Autodesk Inventor part; units mm, degrees
ref_plane "YZ Plane" through (0, 0, 0) normal (1, 0, 0) x (0, 1, 0)
ref_plane "XZ Plane" through (0, 0, 0) normal (0, 1, 0) x (-1, 0, 0)
ref_plane "XY Plane" through (0, 0, 0) normal (0, 0, 1) x (1, 0, 0)
sketch "Sketch1" plane through (0, 0, 0) normal (0, 0, 1) x (1, 0, 0)
  line L0 (-8.2268, 11.9764) -> (-8.2268, -9.0421)
  line L1 (-8.2268, -9.0421) -> (4.4732, -9.0421)
  line L2 (4.4732, -9.0421) -> (4.4732, 11.9764)
  line L3 (4.4732, 11.9764) -> (1.2982, 11.9764)
  line L4 (-8.2268, 11.9764) -> (-5.0518, 11.9764)
  line L5 (-5.0518, 11.9764) -> (-5.0518, 11.5954)
  line L6 (1.2982, 11.9764) -> (1.2982, 11.5954)
  arc A0 (-5.0518, 11.5954) -> (1.2982, 11.5954) centre (-1.8768, 11.5954) ccw
  dimension "d0" = 3.175
  dimension "d1" = 12.7
  dimension "d2" = 0.381
  dimension "d5" = 20.6375
  dimension "d6" = 3.175
  dimension "d7" = 21.0185
revolve "Revolution1" add sketch "Sketch1" angle 360 about axis through (-8.2268, -9.0421, 0) along (1, 0, 0)
sketch "Sketch2" plane through (4.4732, -9.0421, 0) normal (1, 0, 0) x (0, 0, -1)
  circle A0 centre (0, 0) radius 21.0185
hole "Hole1" at (4.4732, -9.0421, 0) direction (-1, 0, 0) diameter 9.525 end through all
sketch "Sketch3" plane through (4.4732, -9.0421, 0) normal (1, 0, 0) x (0, 0, -1)
  circle A0 centre (0, 0) radius 4.7625
  circle A1 centre (0, 0) radius 21.0185
  circle A2 centre (0, 0) radius 4.7625
  circle A3 centre (0, 0) radius 7.9375
  dimension "d15" = 3.175
extrude "Extrusion1" add sketch "Sketch3" along normal blind 12.7 contours A3
properties part number "pulley 1.5"
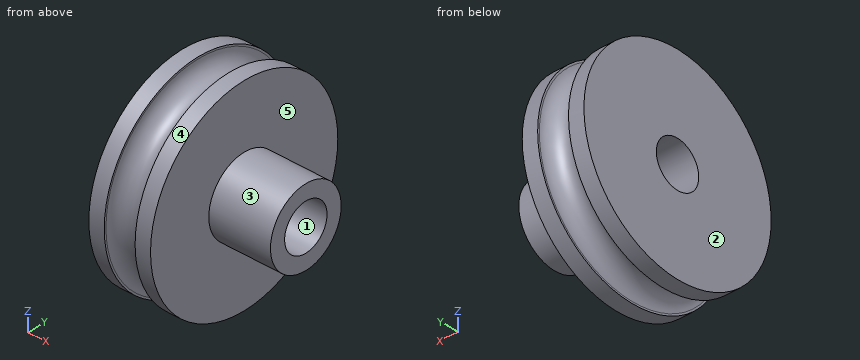
Read the model definition and answer for the solid it produces. Units are mm, in the model's axes. Face numbers are marked on the shaded views. A direction names the side the tool comes from. Round coordinates to 2 decimals unless told otherwise and drop trailing zeros. Write each loop counter-clockwise with the first axis right and the second up, starting at its lowest first coordinate (ties: lowest second). Pieces come first, ordered by that corner, then holes.
1. The part is cut by section A-A, the plane z = 0. Determine the outline of the cut face in (x, y) (3 decimals), then the cut area to 3 significant figures.
2. Straight lines are drawn through the part: L1, parallel to X at y = 1, z = 18; L2, parallel to X at y = -19, z = 8; L3, parallel to Y at x = 8.5, z = 0. For each, find the intervals that lie inside material, in ascending order.
3. Determine the mould class of the marked faces 1, 2 and 3 for opening direction Y: pulls with the +Y half, pulls with the -Y half, needs draft (parallel to the pull), parting line crosses it, or undercut.
4. The part is cut by section C-C, the plane x = 3.5. Determine the outline of the cut face in (y, z) (1 decimal), then the cut area to 3 significant figures.
5. The part is cut by section B-B, the plane x = 14.75. Determine the outline of the cut face in (y, z) (1 decimal).
6. Which of the six approach directions +Z, -Z, +X, -X, +Y, -Y give full straight-line access (tool end or side, diameter ignored) to the marked faces 4 and 5?
7. Given pin 1 Ø5 at (y, z) = (4.5, 16.5) entering from +X; pin 2 Ø5 at (x, y) = (12, -16.5) entering from -Z; pin 3 Ø1 at (x, y) = (3.5, 2.5) entering from -Z, each flat-ended and moving along its own axis, determine where each tip first touches the part or whether it passes through.
Values:
1. outline: (-8.227, -30.061) - (-5.052, -30.061) - (-5.052, -29.68) arc R3.175 cw to (1.298, -29.68) - (1.298, -30.061) - (4.473, -30.061) - (4.473, -16.98) - (17.173, -16.98) - (17.173, -13.805) - (-8.227, -13.805) - close; (-8.227, -4.28) - (17.173, -4.28) - (17.173, -1.105) - (4.473, -1.105) - (4.473, 11.976) - (1.298, 11.976) - (1.298, 11.595) arc R3.175 cw to (-5.052, 11.595) - (-5.052, 11.976) - (-8.227, 11.976) - close
1. area: 457 mm2
2. L1: x = -8.23 to -5.05, 1.3 to 4.47
2. L2: x = -8.23 to 4.47
2. L3: y = -16.98 to -13.8, -4.28 to -1.1
3. face 1: undercut
3. face 2: needs draft
3. face 3: parting line crosses it
4. outline: circle Ø42 at (-9, 0); hole circle Ø9.5 at (-9, 0)
4. area: 1,320 mm2
5. outline: circle Ø15.9 at (-9, 0); hole circle Ø9.5 at (-9, 0)
6. face 4: +X, -X
6. face 5: +X
7. pin 1: stops at x = 4.47
7. pin 2: stops at z = -6.2
7. pin 3: stops at z = -17.88
